from build123d import *

# Parameters (mm, degrees)
SKETCH2_R           = 14.225
SKETCH2_R_2         = 3.18
SKETCH2_R_3         = 1.25
BOSS_EXTRUDE1_DEPTH = 4.7625


with BuildPart() as part:
    # Sketch2 → Boss-Extrude1 (new body)
    with BuildSketch(Plane(origin=(0, 0, 0), x_dir=(0, 0, -1), z_dir=(1, 0, 0))):
        with BuildLine():
            Line((-23.48132736, 28.668303571), (-23.48132736, -31.331696429))
            ThreePointArc((-23.48132736, -31.331696429), (-20.552395172, -38.40276424), (-13.48132736, -41.331696429))
            Line((-13.48132736, -41.331696429), (376.51867264, -41.331696429))
            ThreePointArc((376.51867264, -41.331696429), (383.589740452, -38.40276424), (386.51867264, -31.331696429))
            Line((386.51867264, -31.331696429), (386.51867264, 28.668303571))
            ThreePointArc((386.51867264, 28.668303571), (383.589740452, 35.739371383), (376.51867264, 38.668303571))
            Line((376.51867264, 38.668303571), (-13.48132736, 38.668303571))
            ThreePointArc((-13.48132736, 38.668303571), (-20.552395172, 35.739371383), (-23.48132736, 28.668303571))
        make_face()
        with Locations(Location((29.51867264, -16.331696429, 0), (0, 0, 180))):
            Circle(SKETCH2_R, mode=Mode.SUBTRACT)
        with Locations(Location((333.51867264, -16.331696429, 0), (0, 0, 180))):
            Circle(SKETCH2_R, mode=Mode.SUBTRACT)
        with Locations(Location((181.51867264, -28.771696429, 0), (0, 0, 180))):
            Circle(SKETCH2_R_2, mode=Mode.SUBTRACT)
        with Locations(Location((197.51867264, -28.771696429, 0), (0, 0, 180))):
            Circle(SKETCH2_R_2, mode=Mode.SUBTRACT)
        with Locations(Location((197.51867264, 19.228303571, 0), (0, 0, 180))):
            Circle(SKETCH2_R_2, mode=Mode.SUBTRACT)
        with Locations(Location((181.51867264, -12.771696429, 0), (0, 0, 180))):
            Circle(SKETCH2_R_2, mode=Mode.SUBTRACT)
        with Locations(Location((181.51867264, 3.228303571, 0), (0, 0, 180))):
            Circle(SKETCH2_R_2, mode=Mode.SUBTRACT)
        with Locations(Location((181.51867264, 19.228303571, 0), (0, 0, 180))):
            Circle(SKETCH2_R_2, mode=Mode.SUBTRACT)
        with Locations(Location((165.51867264, -28.771696429, 0), (0, 0, 180))):
            Circle(SKETCH2_R_2, mode=Mode.SUBTRACT)
        with Locations(Location((165.51867264, 19.228303571, 0), (0, 0, 180))):
            Circle(SKETCH2_R_2, mode=Mode.SUBTRACT)
        with Locations(Location((1.51867264, 31.168303571, 0), (0, 0, 180))):
            Circle(SKETCH2_R_3, mode=Mode.SUBTRACT)
        with Locations(Location((11.51867264, 31.168303571, 0), (0, 0, 180))):
            Circle(SKETCH2_R_3, mode=Mode.SUBTRACT)
        with Locations(Location((21.51867264, 31.168303571, 0), (0, 0, 180))):
            Circle(SKETCH2_R_3, mode=Mode.SUBTRACT)
        with Locations(Location((31.51867264, 31.168303571, 0), (0, 0, 180))):
            Circle(SKETCH2_R_3, mode=Mode.SUBTRACT)
        with Locations(Location((41.51867264, 31.168303571, 0), (0, 0, 180))):
            Circle(SKETCH2_R_3, mode=Mode.SUBTRACT)
        with Locations(Location((51.51867264, 31.168303571, 0), (0, 0, 180))):
            Circle(SKETCH2_R_3, mode=Mode.SUBTRACT)
        with Locations(Location((61.51867264, 31.168303571, 0), (0, 0, 180))):
            Circle(SKETCH2_R_3, mode=Mode.SUBTRACT)
        with Locations(Location((71.51867264, 31.168303571, 0), (0, 0, 180))):
            Circle(SKETCH2_R_3, mode=Mode.SUBTRACT)
        with Locations(Location((81.51867264, 31.168303571, 0), (0, 0, 180))):
            Circle(SKETCH2_R_3, mode=Mode.SUBTRACT)
        with Locations(Location((91.51867264, 31.168303571, 0), (0, 0, 180))):
            Circle(SKETCH2_R_3, mode=Mode.SUBTRACT)
        with Locations(Location((101.51867264, 31.168303571, 0), (0, 0, 180))):
            Circle(SKETCH2_R_3, mode=Mode.SUBTRACT)
        with Locations(Location((111.51867264, 31.168303571, 0), (0, 0, 180))):
            Circle(SKETCH2_R_3, mode=Mode.SUBTRACT)
        with Locations(Location((121.51867264, 31.168303571, 0), (0, 0, 180))):
            Circle(SKETCH2_R_3, mode=Mode.SUBTRACT)
        with Locations(Location((131.51867264, 31.168303571, 0), (0, 0, 180))):
            Circle(SKETCH2_R_3, mode=Mode.SUBTRACT)
        with Locations(Location((141.51867264, 31.168303571, 0), (0, 0, 180))):
            Circle(SKETCH2_R_3, mode=Mode.SUBTRACT)
        with Locations(Location((151.51867264, 31.168303571, 0), (0, 0, 180))):
            Circle(SKETCH2_R_3, mode=Mode.SUBTRACT)
        with Locations(Location((161.51867264, 31.168303571, 0), (0, 0, 180))):
            Circle(SKETCH2_R_3, mode=Mode.SUBTRACT)
        with Locations(Location((171.51867264, 31.168303571, 0), (0, 0, 180))):
            Circle(SKETCH2_R_3, mode=Mode.SUBTRACT)
        with Locations(Location((181.51867264, 31.168303571, 0), (0, 0, 180))):
            Circle(SKETCH2_R_3, mode=Mode.SUBTRACT)
        with Locations(Location((191.51867264, 31.168303571, 0), (0, 0, 180))):
            Circle(SKETCH2_R_3, mode=Mode.SUBTRACT)
        with Locations(Location((201.51867264, 31.168303571, 0), (0, 0, 180))):
            Circle(SKETCH2_R_3, mode=Mode.SUBTRACT)
        with Locations(Location((211.51867264, 31.168303571, 0), (0, 0, 180))):
            Circle(SKETCH2_R_3, mode=Mode.SUBTRACT)
        with Locations(Location((221.51867264, 31.168303571, 0), (0, 0, 180))):
            Circle(SKETCH2_R_3, mode=Mode.SUBTRACT)
        with Locations(Location((231.51867264, 31.168303571, 0), (0, 0, 180))):
            Circle(SKETCH2_R_3, mode=Mode.SUBTRACT)
        with Locations(Location((241.51867264, 31.168303571, 0), (0, 0, 180))):
            Circle(SKETCH2_R_3, mode=Mode.SUBTRACT)
        with Locations(Location((251.51867264, 31.168303571, 0), (0, 0, 180))):
            Circle(SKETCH2_R_3, mode=Mode.SUBTRACT)
        with Locations(Location((261.51867264, 31.168303571, 0), (0, 0, 180))):
            Circle(SKETCH2_R_3, mode=Mode.SUBTRACT)
        with Locations(Location((271.51867264, 31.168303571, 0), (0, 0, 180))):
            Circle(SKETCH2_R_3, mode=Mode.SUBTRACT)
        with Locations(Location((281.51867264, 31.168303571, 0), (0, 0, 180))):
            Circle(SKETCH2_R_3, mode=Mode.SUBTRACT)
        with Locations(Location((291.51867264, 31.168303571, 0), (0, 0, 180))):
            Circle(SKETCH2_R_3, mode=Mode.SUBTRACT)
        with Locations(Location((301.51867264, 31.168303571, 0), (0, 0, 180))):
            Circle(SKETCH2_R_3, mode=Mode.SUBTRACT)
        with Locations(Location((311.51867264, 31.168303571, 0), (0, 0, 180))):
            Circle(SKETCH2_R_3, mode=Mode.SUBTRACT)
        with Locations(Location((321.51867264, 31.168303571, 0), (0, 0, 180))):
            Circle(SKETCH2_R_3, mode=Mode.SUBTRACT)
        with Locations(Location((331.51867264, 31.168303571, 0), (0, 0, 180))):
            Circle(SKETCH2_R_3, mode=Mode.SUBTRACT)
        with Locations(Location((341.51867264, 31.168303571, 0), (0, 0, 180))):
            Circle(SKETCH2_R_3, mode=Mode.SUBTRACT)
        with Locations(Location((351.51867264, 31.168303571, 0), (0, 0, 180))):
            Circle(SKETCH2_R_3, mode=Mode.SUBTRACT)
        with Locations(Location((361.51867264, 31.168303571, 0), (0, 0, 180))):
            Circle(SKETCH2_R_3, mode=Mode.SUBTRACT)
        with Locations(Location((101.51867264, -33.831696429, 0), (0, 0, 180))):
            Circle(SKETCH2_R_3, mode=Mode.SUBTRACT)
        with Locations(Location((261.51867264, -33.831696429, 0), (0, 0, 180))):
            Circle(SKETCH2_R_3, mode=Mode.SUBTRACT)
        with Locations(Location((-13.48132736, 28.668303571, 0), (0, 0, 180))):
            Circle(SKETCH2_R_2, mode=Mode.SUBTRACT)
        with Locations(Location((376.51867264, 28.668303571, 0), (0, 0, 180))):
            Circle(SKETCH2_R_2, mode=Mode.SUBTRACT)
        with Locations(Location((101.51867264, -17.581696429, 0), (0, 0, 180))):
            Circle(SKETCH2_R_3, mode=Mode.SUBTRACT)
        with Locations(Location((261.51867264, -17.581696429, 0), (0, 0, 180))):
            Circle(SKETCH2_R_3, mode=Mode.SUBTRACT)
        with Locations(Location((101.51867264, -1.331696429, 0), (0, 0, 180))):
            Circle(SKETCH2_R_3, mode=Mode.SUBTRACT)
        with Locations(Location((261.51867264, -1.331696429, 0), (0, 0, 180))):
            Circle(SKETCH2_R_3, mode=Mode.SUBTRACT)
        with Locations(Location((101.51867264, 14.918303571, 0), (0, 0, 180))):
            Circle(SKETCH2_R_3, mode=Mode.SUBTRACT)
        with Locations(Location((261.51867264, 14.918303571, 0), (0, 0, 180))):
            Circle(SKETCH2_R_3, mode=Mode.SUBTRACT)
    extrude(amount=BOSS_EXTRUDE1_DEPTH)


solid = part.part
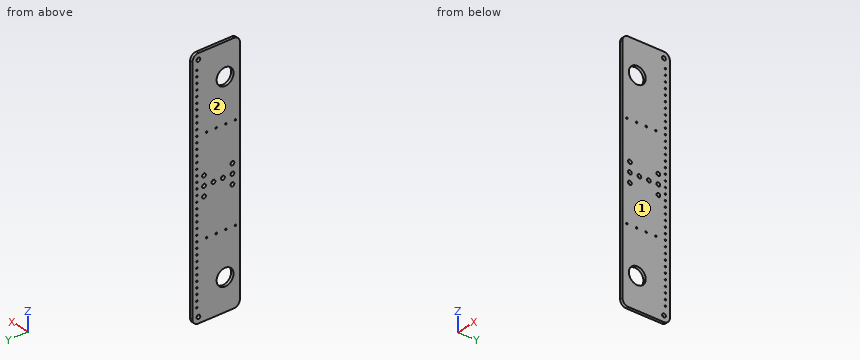
Here's how the part is built. I have some questions about the finished solid (model axes, mm). Face numbers are marked on the shaded views. Coordinates: 2 decimals unless noted, no trailing zeros.
Item 1: I need wall thicknesses on line 1 (Y direction, x = 0.7, z = -165.5); line 2 (Y direction, x = 0.9, z = -197); line 3 (Z direction, x = 4.2, y = 3.5). Which ranges of each line are inside material? Lowest first, please.
Result sheet:
line 1: y = -41.33 to -31.95, -25.59 to 16.05, 22.41 to 38.67
line 2: y = -41.33 to -31.91, -25.63 to 16.09, 22.37 to 38.67
line 3: z = -386.52 to -184.69, -178.35 to 23.48
Item 2: If we mould it in two halves opening along X, with no side actions, what happens to the marked faces 1 and 2? For each: +X half, -X half, draft (parallel to the pull), parting line (faces both ways), or undercut.
Result sheet:
face 1: +X half
face 2: -X half
Item 3: For P1, Ø2, axis at y = 31.17, z = -151.52, coming from the +X side, with a flat end and sliding along its axis, tell me the tip position at first contact or that it passes through.
Result sheet:
P1: passes through
Item 4: If we section it at A-A on x = 3.2: State how many separate pieces and enclosed holes the cut face has, plus the area to 3 significant figures.
Result sheet:
separate pieces: 1
enclosed holes: 57
area: 30,900 mm2
